from build123d import *

# Parameters (mm, degrees)
SKETCH1_R                      = 0.005
BOSS_EXTRUDE1_DEPTH            = 0.003
SKETCH2_R                      = 0.0079
SKETCH2_R_2                    = 0.004201919
BOSS_EXTRUDE3_DEPTH            = 0.01
CHAMFER1_SIZE                  = 0.0005
CUT_EXTRUDE1_REACH             = 2.054
SKETCH3_R                      = 0.00085
CUT_EXTRUDE1_DIRECTION_2_DEPTH = 1.053763073
CIRPATTERN1_COUNT              = 3
SCALE1_SCALE                   = 1000


with BuildPart() as part:
    # Sketch1 → Boss-Extrude1 (new body)
    with BuildSketch(Plane.XY):
        with BuildLine():
            Line((0.009008368, -0.025787204), (-0.009991632, -0.025787204))
            ThreePointArc((-0.009991632, -0.025787204), (-0.013527166, -0.02725167), (-0.014991632, -0.030787204))
            Line((-0.014991632, -0.030787204), (-0.014991632, -0.040787204))
            ThreePointArc((-0.014991632, -0.040787204), (-0.013527166, -0.044322738), (-0.009991632, -0.045787204))
            Line((-0.009991632, -0.045787204), (0.009008368, -0.045787204))
            ThreePointArc((0.009008368, -0.045787204), (0.009715474, -0.045494311), (0.010008368, -0.044787204))
            Line((0.010008368, -0.044787204), (0.010008368, -0.026787204))
            ThreePointArc((0.010008368, -0.026787204), (0.009715474, -0.026080097), (0.009008368, -0.025787204))
        make_face()
        with Locations((0, -0.035787204)):
            Circle(SKETCH1_R, mode=Mode.SUBTRACT)
    extrude(amount=BOSS_EXTRUDE1_DEPTH)

    # Sketch2 → Boss-Extrude3 (add)
    with BuildSketch(Plane.XY.offset(0.003)):
        with Locations((0, -0.035787204)):
            Circle(SKETCH2_R)
        with Locations((0, -0.035787204)):
            Circle(SKETCH2_R_2, mode=Mode.SUBTRACT)
    extrude(amount=BOSS_EXTRUDE3_DEPTH)

    # Chamfer1
    chamfer1_edges = [part.edges().sort_by_distance(p)[0] for p in [
        (-0.000491632, -0.045787204, 0),
        (-0.013527166, -0.044322738, 0),
        (-0.014991632, -0.035787204, 0),
        (0.009715474, -0.045494311, 0.003),
        (-0.013527166, -0.02725167, 0),
        (-0.000491632, -0.025787204, 0),
        (0.009715474, -0.026080097, 0),
        (0.010008368, -0.035787204, 0),
        (0.009715474, -0.045494311, 0),
        (-0.005, -0.035787204, 0),
        (0.010008368, -0.035787204, 0.003),
        (0.009715474, -0.026080097, 0.003),
        (-0.000491632, -0.025787204, 0.003),
        (-0.0079, -0.035787204, 0.003),
        (-0.013527166, -0.02725167, 0.003),
        (-0.0079, -0.035787204, 0.013),
        (-0.004201919, -0.035787204, 0.013),
        (-0.014991632, -0.035787204, 0.003),
        (-0.013527166, -0.044322738, 0.003),
        (-0.000491632, -0.045787204, 0.003),
    ]]
    chamfer(chamfer1_edges, length=CHAMFER1_SIZE)

    # Sketch3 → Cut-Extrude1 (cut, up to next)
    with BuildSketch(Plane(origin=(0.010008368, 0, 0), x_dir=(0, 0, -1), z_dir=(1, 0, 0)), mode=Mode.PRIVATE) as cut_extrude1_sk1:
        with Locations(Location((-0.008204866, -0.035787204, 0), (0, 0, 90))):
            Circle(SKETCH3_R)
    cut_extrude1_tool1 = extrude(cut_extrude1_sk1.sketch, amount=-CUT_EXTRUDE1_REACH, mode=Mode.PRIVATE) & part.part
    cut_extrude1 = cut_extrude1_tool1.solids().sort_by_distance((0.010008, -0.035787, 0.008205))[0]
    add(cut_extrude1, mode=Mode.SUBTRACT)

    # Sketch3 → Cut-Extrude1 direction 2 (cut)
    with BuildSketch(Plane(origin=(0.010008368, 0, 0), x_dir=(0, 0, -1), z_dir=(1, 0, 0))):
        with Locations(Location((-0.008204866, -0.035787204, 0), (0, 0, 90))):
            Circle(SKETCH3_R)
    cut_extrude1_direction_2 = extrude(amount=CUT_EXTRUDE1_DIRECTION_2_DEPTH, mode=Mode.SUBTRACT)

    # CirPattern1: Cut-Extrude1, Cut-Extrude1 direction 2 ×3 about axis
    cirpattern1_axis = Axis((0, -0.035787204, 0.0125), (0, 0, 1))
    add([cut_extrude1.rotate(cirpattern1_axis, i * 360 / CIRPATTERN1_COUNT) for i in range(1, CIRPATTERN1_COUNT)], mode=Mode.SUBTRACT)
    add([cut_extrude1_direction_2.rotate(cirpattern1_axis, i * 360 / CIRPATTERN1_COUNT) for i in range(1, CIRPATTERN1_COUNT)], mode=Mode.SUBTRACT)


with BuildPart() as part_1:
    # Scale1: scaled about (-0.001262886, -0.035787205, 0.004936409)
    add(part.part.scale(SCALE1_SCALE).moved(Location((1.261623114, 35.751417795, -4.931472591))))


solid = part_1.part
Geometry check sheet. Reference: the model listing, model coordinates, mm. A direction names the side the tool comes from. Give positions to 0.01 mm unless a question says otherwise; leave off trailing zeros. Loops run counter-clockwise (first coordinate to the right, second up) from the corner with the lowest first, then second, coordinate; pieces in that order, holes last. Notation, with made-up numbers: M 48.5,3.5 L 106.5,3.5 A21 cw 106.5,7.5 Z; hole C 70,16 d2. An arc over 180 degrees is marked long. Write each question's results on one line, items separated by ' | '.
1) Section check A-A, the plane x = -8.25. Record the boundary of the cut face in (y, z).
Answers follow:
outline: M -10.04,-4.43 L -9.54,-4.93 L 9.46,-4.93 L 9.96,-4.43 L 9.96,-2.43 L 9.46,-1.93 L -9.54,-1.93 L -10.04,-2.43 Z
2) Gauge pin test, flat ends, axial feed: pin 1 (6 mm diameter, centred on x = 5, z = 2.5, fed in from +Y); pin 2 (2 mm diameter, centred on y = -0.04, z = 3.27, fed in from -X); pin 3 (1.5 mm diameter, centred on y = 4, z = 5.5, fed in from -X). Record the tip position at first contact, or that the pin passes through.
Answers follow:
pin 1: y = 7.83 | pin 2: x = -6.64 | pin 3: x = -5.92
3) Tool access check on faces 1 (the face through (-13.73, 0, -3)), 2 (the face through (7.3, -0.66, 3.85)), 3 (the face through (-7, 4, -1.931)). Record the directions out of +Z, -Z, +X, -X, +Y, -Y that give a thin tool (end or side, any length) a straight path to the whole face; none if there is none.
Answers follow:
face 1: +Z, -Z, -X, +Y, -Y | face 2: +X | face 3: +Z
4) Thickness scan on line 1 (Y direction, x = 1.5, z = 5.5); line 2 (X direction, y = 0, z = 1); line 3 (Z direction, x = 10, y = -0.25). Record the ranges inside material, lowest first.
Answers follow:
line 1: -7.93 to -4.23, 4.16 to 7.86 | line 2: -6.64 to -2.94, 5.46 to 9.16 | line 3: -4.93 to -1.93
5) Release check for a two-part mould opening along X. For faces 4 (the face through (-2, 3, -1.931)), 5 (the face through (-11.971, 8.278, -4.796)), 6 (the face through (11.27, 0, -3)) record: +X half, -X half, draft (parallel to the pull), parting line (faces both ways), or undercut.
Answers follow:
face 4: undercut | face 5: -X half | face 6: +X half
6) Section check B-B, the plane z = 5.75. Record the boundary of the cut face in (x, y).
Answers follow:
outline: C 1.26,-0.04 d15.8; hole C 1.26,-0.04 d8.4
